Can you work these out from the model? Positions are in its coordinate system, mm. A direction names the side the tool comes from. Round coordinates to 2 decimals unless told otherwise and drop trailing zeros. Loops run counter-clockwise (first coordinate to the right, second up) from the corner with the lowest first, then second, coordinate; pieces in that order, holes last.
from build123d import *

# Parameters (mm, degrees)
CROQUIS1_R              = 43.5
CROQUIS1_R_2            = 30
SALIENTE_EXTRUIR1_DEPTH = 4
CROQUIS2_R              = 30
CROQUIS2_R_2            = 20
SALIENTE_EXTRUIR2_DEPTH = 4
CROQUIS3_R              = 30
CROQUIS3_R_2            = 20
CORTAR_EXTRUIR1_DEPTH   = 2
CROQUIS5_R              = 3
CORTAR_EXTRUIR3_DEPTH   = 4
SALIENTE_EXTRUIR3_DEPTH = 200
CROQUIS8_R              = 45.5
SALIENTE_EXTRUIR4_DEPTH = 4
CROQUIS9_R              = 21
CROQUIS9_R_2            = 19
SALIENTE_EXTRUIR5_DEPTH = 33
CORTAR_EXTRUIR6_START   = -33
CORTAR_EXTRUIR6_DEPTH   = 33
CROQUIS11_R             = 21
SALIENTE_EXTRUIR6_DEPTH = 4
CORTAR_EXTRUIR7_START   = -4
CORTAR_EXTRUIR7_DEPTH   = 4
CROQUIS14_R             = 45.5
CORTAR_EXTRUIR9_DEPTH   = 4
CORTAR_EXTRUIR11_DEPTH  = 200
CROQUIS16_R             = 10
CORTAR_EXTRUIR12_DEPTH  = 4
CORTAR_EXTRUIR13_START  = 200
CORTAR_EXTRUIR13_DEPTH  = 4


with BuildPart() as part:
    # Croquis1 → Saliente-Extruir1 (new body)
    with BuildSketch(Plane(origin=(0, 0, 0), x_dir=(1, 0, 0), z_dir=(0, 1, 0))):
        with Locations(Location((0, 0, 0), (0, 0, 270))):
            Circle(CROQUIS1_R)
        with Locations(Location((0, 0, 0), (0, 0, 270))):
            Circle(CROQUIS1_R_2, mode=Mode.SUBTRACT)
    extrude(amount=SALIENTE_EXTRUIR1_DEPTH)

    # Croquis2 → Saliente-Extruir2 (add)
    with BuildSketch(Plane(origin=(0, 0, 0), x_dir=(1, 0, 0), z_dir=(0, 1, 0))):
        Circle(CROQUIS2_R)
        with Locations(Location((0, 0, 0), (0, 0, 270))):
            Circle(CROQUIS2_R_2, mode=Mode.SUBTRACT)
    extrude(amount=SALIENTE_EXTRUIR2_DEPTH)

    # Croquis3 → Cortar-Extruir1 (cut)
    with BuildSketch(Plane(origin=(0, 0, 0), x_dir=(1, 0, 0), z_dir=(0, 1, 0))):
        with Locations(Location((0, 0, 0), (0, 0, 270))):
            Circle(CROQUIS3_R)
        with Locations(Location((0, 0, 0), (0, 0, 270))):
            Circle(CROQUIS3_R_2, mode=Mode.SUBTRACT)
    extrude(amount=CORTAR_EXTRUIR1_DEPTH, mode=Mode.SUBTRACT)

    # Croquis5 → Cortar-Extruir3 (cut)
    with BuildSketch(Plane(origin=(0, 0, 0), x_dir=(1, 0, 0), z_dir=(0, 1, 0))):
        with Locations(Location((0, -37.5, 0), (0, 0, 270))):
            Circle(CROQUIS5_R)
        with Locations(Location((-37.5, 0, 0), (0, 0, 270))):
            Circle(CROQUIS5_R)
        with Locations(Location((0, 37.5, 0), (0, 0, 270))):
            Circle(CROQUIS5_R)
        with Locations(Location((37.5, 0, 0), (0, 0, 270))):
            Circle(CROQUIS5_R)
    extrude(amount=CORTAR_EXTRUIR3_DEPTH, mode=Mode.SUBTRACT)

    # Croquis7 → Saliente-Extruir3 (add)
    with BuildSketch(Plane(origin=(0, 0, 0), x_dir=(1, 0, 0), z_dir=(0, 1, 0))):
        with BuildLine():
            Line((-45.5, 0), (-43.5, 0))
            ThreePointArc((-43.5, 0), (0, -43.5), (43.5, 0))
            Line((43.5, 0), (45.5, 0))
            ThreePointArc((45.5, 0), (0, -45.5), (-45.5, 0))
        make_face()
    extrude(amount=SALIENTE_EXTRUIR3_DEPTH)

    # Croquis8 → Saliente-Extruir4 (add)
    with BuildSketch(Plane(origin=(0, 200, 0), x_dir=(1, 0, 0), z_dir=(0, 1, 0))):
        Circle(CROQUIS8_R)
    extrude(amount=SALIENTE_EXTRUIR4_DEPTH)

    # Croquis9 → Saliente-Extruir5 (add)
    with BuildSketch(Plane.XZ.offset(-200)):
        with Locations(Location((0, 0, 0), (0, 0, 90))):
            Circle(CROQUIS9_R)
        with Locations(Location((0, 0, 0), (0, 0, 270))):
            Circle(CROQUIS9_R_2, mode=Mode.SUBTRACT)
    extrude(amount=SALIENTE_EXTRUIR5_DEPTH)

    # Croquis10 → Cortar-Extruir6 (cut)
    with BuildSketch(Plane.XZ.offset(-167).offset(CORTAR_EXTRUIR6_START)):
        with BuildLine():
            Line((21, 0), (-21, 0))
            ThreePointArc((-21, 0), (0, -21), (21, 0))
        make_face()
    extrude(amount=CORTAR_EXTRUIR6_DEPTH, mode=Mode.SUBTRACT)

    # Croquis11 → Saliente-Extruir6 (add)
    with BuildSketch(Plane.XZ.offset(-167)):
        with Locations(Location((0, 0, 0), (0, 0, 180))):
            Circle(CROQUIS11_R)
    extrude(amount=SALIENTE_EXTRUIR6_DEPTH)

    # Croquis12 → Cortar-Extruir7 (cut)
    with BuildSketch(Plane.XZ.offset(-163).offset(CORTAR_EXTRUIR7_START)):
        with BuildLine():
            Line((-3, 0), (-3, -20.784609691))
            ThreePointArc((-3, -20.784609691), (0, -21), (3, -20.784609691))
            Line((3, -20.784609691), (3, 0))
            ThreePointArc((3, 0), (0, 3), (-3, 0))
        make_face()
    extrude(amount=CORTAR_EXTRUIR7_DEPTH, mode=Mode.SUBTRACT)

    # Croquis14 → Cortar-Extruir9 (cut)
    with BuildSketch(Plane.XZ):
        Circle(CROQUIS14_R)
    extrude(amount=-CORTAR_EXTRUIR9_DEPTH, mode=Mode.SUBTRACT)

    # Croquis15 → Cortar-Extruir11 (cut)
    with BuildSketch(Plane(origin=(0, 0, 0), x_dir=(1, 0, 0), z_dir=(0, 1, 0))):
        with BuildLine():
            Line((43.5, 0), (45.5, 0))
            ThreePointArc((45.5, 0), (32.173358544, -32.173358544), (0, -45.5))
            Line((0, -45.5), (0, -43.5))
            ThreePointArc((0, -43.5), (30.759144982, -30.759144982), (43.5, 0))
        make_face()
    extrude(amount=CORTAR_EXTRUIR11_DEPTH, mode=Mode.SUBTRACT)

    # Croquis16 → Cortar-Extruir12 (cut)
    with BuildSketch(Plane.XZ.offset(-163)):
        Circle(CROQUIS16_R)
    extrude(amount=-CORTAR_EXTRUIR12_DEPTH, mode=Mode.SUBTRACT)

    # Croquis17 → Cortar-Extruir13 (cut)
    with BuildSketch(Plane(origin=(0, 0, 0), x_dir=(1, 0, 0), z_dir=(0, 1, 0)).offset(CORTAR_EXTRUIR13_START)):
        with BuildLine():
            Line((-45.5, 0), (45.5, 0))
            ThreePointArc((45.5, 0), (0, 45.5), (-45.5, 0))
        make_face()
    extrude(amount=CORTAR_EXTRUIR13_DEPTH, mode=Mode.SUBTRACT)


solid = part.part
(1) If we section it at A-A, the plane x = 6: List the corners of the cut face in (y, z) for me.
Worked answers:
outline: (163, -20.12) - (167, -20.12) - (167, -8) - (163, -8) - close; (163, 8) - (167, 8) - (167, 18.03) - (200, 18.03) - (200, 0) - (204, 0) - (204, 45.1) - (200, 45.1) - (200, 20.12) - (163, 20.12) - close
(2) For faces 1 (the flat face through (3, 165, -15)), 2 (the flat face through (-9, 167, -6)), 3 (the flat face through (0, 200, 22)), which set-ups out of +Z, -Z, +X, -X, +Y, -Y let a thin tool reach every point of the face, with its end or its side?
Worked answers:
face 1: -Z, +Y, -Y
face 2: -Z
face 3: -Y
(3) Will these pins go through, and if not, where does the flat tip stop? P1, Ø6, axis at x = 15.5, z = -1.5, coming from the -Y side; P2, Ø12, axis at x = 0, z = 0, coming from the -Y side; P3, Ø1.5, axis at x = 11.5, y = 171.5, coming from the -Z side.
Worked answers:
P1: stops at y = 163
P2: stops at y = 200
P3: stops at z = 14.52
(4) If we section it at D-D, the plane y = 34: List the corners of the cut face in (x, z) for me, then the cut area to 3 significant figures.
Worked answers:
outline: (-45.5, 0) - (-43.5, 0) arc R43.5 cw to (0, 43.5) - (0, 45.5) arc R45.5 ccw to start
area: 140 mm2
(5) If I drill on line 1 (Y direction, x = -6, z = 15); line 2 (X direction, y = 169.5, z = 14); line 3 (Y direction, x = 15, z = -7.5), over which ranges is the centre line in solid material (lowest first)?
Worked answers:
line 1: y = 163 to 167, 200 to 204
line 2: x = -43.29 to -41.19, -15.65 to -12.85, 12.85 to 15.65
line 3: y = 163 to 167
(6) If we section it at C-C, the plane z = 16: List the corners of the cut face in (x, y) for me, then the cut area to 3 significant figures.
Worked answers:
outline: (-42.59, 4) - (-40.45, 4) - (-40.45, 200) - (-13.6, 200) - (-13.6, 163) - (13.6, 163) - (13.6, 200) - (42.59, 200) - (42.59, 204) - (-42.59, 204) - close; hole (-10.25, 167) - (10.25, 167) - (10.25, 200) - (-10.25, 200) - close
area: 1,090 mm2
(7) If we section it at B-B, the plane z = -14.5: List the corners of the cut face in (x, y) for me, then the cut area to 3 significant figures.
Worked answers:
outline: (-15.19, 163) - (-3, 163) - (-3, 167) - (-15.19, 167) - close; (3, 163) - (15.19, 163) - (15.19, 167) - (3, 167) - close
area: 97.5 mm2
(8) If we mould it in two halves opening along X, with no side actions, what happens to faces 4 (the flat face through (-1, 204, 17)), 5 (the flat face through (-3, 165, -15))? For each: released by +X, released by -X, zero draft, split by the parting line, or undercut.
Worked answers:
face 4: zero draft
face 5: undercut
